Verification items for the finished model (mm, model axes). A direction names the side the tool comes from. Round coordinates to 2 decimals unless told otherwise and drop trailing zeros. Order: outer loops, then holes, each group sorted by start corner. A loop starts at its lowest first (then second) coordinate and runs counter-clockwise, first axis right, second up. Notation, with made-up numbers: (6, 33) -> (11, 33) arc R33 cw to (11, 61) -> close; hole circle Ø4 at (70.25, -40). An arc over 180 degrees is marked (long way). Put each result on its own line as item: value.
from build123d import *
from build123d.topology import SkipClean

# Parameters (mm, degrees)
CROQUIS1_R              = 20.1
CROQUIS1_R_2            = 16.7
SALIENTE_EXTRUIR1_DEPTH = 85
CROQUIS2_R              = 20.1
CROQUIS2_R_2            = 16.7
SALIENTE_EXTRUIR2_DEPTH = 42.44
CROQUIS3_R              = 16.7
CORTAR_EXTRUIR1_DEPTH   = 84.497438367
CORTAR_EXTRUIR2_START   = -42.497438367
CROQUIS5_R              = 16.7
CORTAR_EXTRUIR2_DEPTH   = 42.497438367


with BuildPart() as part:
    # Croquis1 → Saliente-Extruir1 (new body)
    with BuildSketch(Plane(origin=(0, 0, 0), x_dir=(0, 0, -1), z_dir=(1, 0, 0))):
        Circle(CROQUIS1_R)
        Circle(CROQUIS1_R_2, mode=Mode.SUBTRACT)
    extrude(amount=SALIENTE_EXTRUIR1_DEPTH)

    # Croquis2 → Saliente-Extruir2 (add)
    with BuildSketch(Plane(origin=(0, 0, 0), x_dir=(1, 0, 0), z_dir=(0, 1, 0))):
        with Locations(Location((42.5, 0, 0), (0, 0, 270))):
            Circle(CROQUIS2_R)
        with Locations(Location((42.5, 0, 0), (0, 0, 90))):
            Circle(CROQUIS2_R_2, mode=Mode.SUBTRACT)
    extrude(amount=SALIENTE_EXTRUIR2_DEPTH)

    # Croquis3 → Cortar-Extruir1 (cut)
    with SkipClean():  # the faces are left unmerged after this step: merging them gives an invalid solid
        with BuildSketch(Plane.ZY):
            with Locations(Location((0, 0, 0), (0, 0, 180))):
                Circle(CROQUIS3_R)
        extrude(amount=-CORTAR_EXTRUIR1_DEPTH, mode=Mode.SUBTRACT)

    # Croquis5 → Cortar-Extruir2 (cut)
    with SkipClean():  # the faces are left unmerged after this step: merging them gives an invalid solid
        with BuildSketch(Plane(origin=(0, 42.44, 0), x_dir=(1, 0, 0), z_dir=(0, 1, 0)).offset(CORTAR_EXTRUIR2_START)):
            with Locations(Location((42.5, 0, 0), (0, 0, 270))):
                Circle(CROQUIS5_R)
        extrude(amount=CORTAR_EXTRUIR2_DEPTH, mode=Mode.SUBTRACT)


solid = part.part
Item 1: Section check A-A on z = 0. Record the boundary of the cut face in (x, y), then the cut area to 3 significant figures.
Check sheet entries:
outline: (0, -20.1) -> (85, -20.1) -> (85, -16.7) -> (0, -16.7) -> close; (0, 16.7) -> (25.8, 16.7) -> (25.8, 42.44) -> (22.4, 42.44) -> (22.4, 20.1) -> (0, 20.1) -> close; (59.2, 16.7) -> (85, 16.7) -> (85, 20.1) -> (62.6, 20.1) -> (62.6, 42.44) -> (59.2, 42.44) -> close
area: 616 mm^2
Item 2: Section check D-D on y = 24. Record the boundary of the cut face in (x, z).
Check sheet entries:
outline: circle Ø40.2 at (42.5, 0); hole circle Ø33.4 at (42.5, 0)
Item 3: Tool access check on faces 4 (the flat face through (0, 15, 8)), 5 (the cylindrical face through (41.905, -17.832, -9.275)). Record the directions out of +Z, -Z, +X, -X, +Y, -Y that give a thin tool (end or side, any length) a straight path to the whole face; none if there is none.
Check sheet entries:
face 4: +Z, -Z, -X, +Y, -Y
face 5: none
Item 4: Section check B-B on y = -3.5. Record the boundary of the cut face in (x, z), then the cut area to 3 significant figures.
Check sheet entries:
outline: (0, -19.79) -> (85, -19.79) -> (85, -16.33) -> (0, -16.33) -> close; (0, 16.33) -> (85, 16.33) -> (85, 19.79) -> (0, 19.79) -> close
area: 589 mm^2
Item 5: Release check for a two-part mould opening along Z. For faces 1 (the cylindrical face through (41.905, -14.816, -7.706)), 2 (the flat face through (85, 15, 8)), 3 (the cylindrical face through (56.1, 25.6, -14.8)) record: +Z half, -Z half, draft (parallel to the pull), parting line (faces both ways), or undercut.
Check sheet entries:
face 1: undercut
face 2: draft
face 3: parting line
Item 6: Material ranges on L1, parallel to X at y = 20.5, z = -0.5; L2, parallel to Y at x = 66.5, z = 0; L3, parallel to Z at x = 42, y = 12, recorded low to high. Write a range as [from, to].
Check sheet entries:
L1: x = [22.41, 25.81], [59.19, 62.59]
L2: y = [-20.1, -16.7], [16.7, 20.1]
L3: z = [-20.09, -16.69], [16.69, 20.09]
Item 7: Section check C-C on x = 80. Record the boundary of the cut face in (y, z), then the cut area to 3 significant figures.
Check sheet entries:
outline: circle Ø40.2 at (0, 0); hole circle Ø33.4 at (0, 0)
area: 393 mm^2
Item 8: Gauge pin test, flat ends, axial feed: pin 1 Ø10 at (x, z) = (68, 7.5) entering from -Y; pin 2 Ø10 at (x, z) = (29.5, -1.5) entering from -Y; pin 3 Ø12 at (x, y) = (34, 6.5) entering from -Z. Record the tip position at first contact, or that the pin passes through.
Check sheet entries:
pin 1: stops at y = -19.94
pin 2: stops at y = -20.1
pin 3: stops at z = -20.09
